Here's how the part is built. I have some questions about the finished solid (model axes, mm). A direction names the side the tool comes from. Give positions to 0.01 mm unless a question says otherwise; leave off trailing zeros. Loops run counter-clockwise (first coordinate to the right, second up) from the corner with the lowest first, then second, coordinate; pieces in that order, holes last.
Q1. Will these pins go through, and if not, where does the flat tip stop? P1, Ø4.5, axis at y = -9.5, z = 4.5, coming from the -X side; P2, Ø3, axis at y = 9, z = 2.5, coming from the +X side; P3, Ø12, axis at x = 8.5, z = 35.5, coming from the -Y side.
Q2. If we section it at C-C (x = -13.5): Please give me the cut outline in (y, z), plus the area to 3 significant figures.
Q3. We'd pull the mould along X, two halves only. Please class faces 1 (the face through (35, -17, 3)), 2 (the face through (-0.6, 5.4, 50)), 3 (the face through (-43, 0, 25)): +X half, -X half, draft (parallel to the pull), parting line (faces both ways), or undercut.
Q4. If we section it at B-B (x = -35): Please give me the cut outline in (y, z), plus the area to 3 significant figures.
Q5. If we section it at D-D (y = -7): Please give me the cut outline in (x, z), plus the area to 3 significant figures.
Q6. I need wall thicknesses on line 1 (X direction, y = -12, z = 3.95); line 2 (Y direction, x = -35, z = 3.6); line 3 (Y direction, x = 14, z = 20.5). Which ranges of each line are inside material? Lowest first, please.
Q7. If we section it at A-A (z = 14): Please give me the cut outline in (x, y), plus the area to 3 significant figures.
Q8. For faces 4 (the face through (-1, -5, 27)), 5 (the face through (-30, 10, 3)), 6 (the face through (40, 10, 3)), which set-ups out of +Z, -Z, +X, -X, +Y, -Y let a thin tool reach every point of the face, with its end or its side?
from build123d import *

# Parameters (mm, degrees)
F0_W     = 80
F0_H     = 10
F1_DEPTH = 50
F2_W     = 80
F2_H     = 10
F3_DEPTH = 5
F4_DEPTH = 6


with BuildPart() as f1:
    # F0 (on Top) → F1 (new body)
    with BuildSketch(Plane.XY):
        with BuildLine():
            ThreePointArc((43, 5), (42.12132, 7.12132), (40, 8))
            Line((40, 8), (30, 8))
            Line((30, 8), (-30, 8))
            Line((-30, 8), (-40, 8))
            ThreePointArc((-40, 8), (-42.12132, 7.12132), (-43, 5))
            Line((-43, 5), (-43, -5))
            ThreePointArc((-43, -5), (-42.12132, -7.12132), (-40, -8))
            Line((-40, -8), (-30, -8))
            Line((-30, -8), (30, -8))
            Line((30, -8), (40, -8))
            ThreePointArc((40, -8), (42.12132, -7.12132), (43, -5))
            Line((43, -5), (43, 5))
        make_face()
        Rectangle(F0_W, F0_H, mode=Mode.SUBTRACT)
    extrude(amount=F1_DEPTH)

    # F2 (on Top) → F3 (join)
    with BuildSketch(Plane.XY):
        Rectangle(F2_W, F2_H)
    extrude(amount=F3_DEPTH)

    # F0 (on Top) → F4 (join)
    with BuildSketch(Plane.XY):
        with BuildLine():
            ThreePointArc((43, 5), (42.12132, 7.12132), (40, 8))
            Line((40, 8), (30, 8))
            Line((30, 8), (-30, 8))
            Line((-30, 8), (-40, 8))
            ThreePointArc((-40, 8), (-42.12132, 7.12132), (-43, 5))
            Line((-43, 5), (-43, -5))
            ThreePointArc((-43, -5), (-42.12132, -7.12132), (-40, -8))
            Line((-40, -8), (-30, -8))
            Line((-30, -8), (30, -8))
            Line((30, -8), (40, -8))
            ThreePointArc((40, -8), (42.12132, -7.12132), (43, -5))
            Line((43, -5), (43, 5))
        make_face()
        Rectangle(F0_W, F0_H, mode=Mode.SUBTRACT)
        with BuildLine():
            Line((30, 8), (40, 8))
            Line((40, 8), (40, 12))
            Line((40, 12), (36.75, 12))
            ThreePointArc((36.75, 12), (35, 10.25), (33.25, 12))
            Line((33.25, 12), (30, 12))
            Line((30, 12), (30, 8))
        make_face()
        with BuildLine():
            Line((36.75, 12), (40, 12))
            ThreePointArc((40, 12), (35, 17), (30, 12))
            Line((30, 12), (33.25, 12))
            ThreePointArc((33.25, 12), (35, 13.75), (36.75, 12))
        make_face()
        with BuildLine():
            Line((-40, 8), (-30, 8))
            Line((-30, 8), (-30, 12))
            Line((-30, 12), (-33.25, 12))
            ThreePointArc((-33.25, 12), (-35, 10.25), (-36.75, 12))
            Line((-36.75, 12), (-40, 12))
            Line((-40, 12), (-40, 8))
        make_face()
        with BuildLine():
            Line((-33.25, 12), (-30, 12))
            ThreePointArc((-30, 12), (-35, 17), (-40, 12))
            Line((-40, 12), (-36.75, 12))
            ThreePointArc((-36.75, 12), (-35, 13.75), (-33.25, 12))
        make_face()
        with BuildLine():
            Line((40, -12), (40, -8))
            Line((40, -8), (30, -8))
            Line((30, -8), (30, -12))
            Line((30, -12), (33.25, -12))
            ThreePointArc((33.25, -12), (35, -10.25), (36.75, -12))
            Line((36.75, -12), (40, -12))
        make_face()
        with BuildLine():
            ThreePointArc((30, -12), (35, -17), (40, -12))
            Line((40, -12), (36.75, -12))
            ThreePointArc((36.75, -12), (35, -13.75), (33.25, -12))
            Line((33.25, -12), (30, -12))
        make_face()
        with BuildLine():
            Line((-30, -12), (-30, -8))
            Line((-30, -8), (-40, -8))
            Line((-40, -8), (-40, -12))
            Line((-40, -12), (-36.75, -12))
            ThreePointArc((-36.75, -12), (-35, -10.25), (-33.25, -12))
            Line((-33.25, -12), (-30, -12))
        make_face()
        with BuildLine():
            ThreePointArc((-40, -12), (-35, -17), (-30, -12))
            Line((-30, -12), (-33.25, -12))
            ThreePointArc((-33.25, -12), (-35, -13.75), (-36.75, -12))
            Line((-36.75, -12), (-40, -12))
        make_face()
    extrude(amount=F4_DEPTH)


solid = f1.part
Check sheet entries:
1. P1: stops at x = -41.98
1. P2: stops at x = 41.66
1. P3: stops at y = -8
2. outline: (-8, 0) - (8, 0) - (8, 50) - (5, 50) - (5, 5) - (-5, 5) - (-5, 50) - (-8, 50) - close
2. area: 350 mm2
3. face 1: undercut
3. face 2: draft
3. face 3: -X half
4. outline: (-17, 0) - (-13.75, 0) - (-13.75, 6) - (-17, 6) - close; (-10.25, 0) - (10.25, 0) - (10.25, 6) - (8, 6) - (8, 50) - (5, 50) - (5, 5) - (-5, 5) - (-5, 50) - (-8, 50) - (-8, 6) - (-10.25, 6) - close; (13.75, 0) - (17, 0) - (17, 6) - (13.75, 6) - close
4. area: 416 mm2
5. outline: (-42.24, 0) - (42.24, 0) - (42.24, 50) - (-42.24, 50) - close
5. area: 4,220 mm2
6. line 1: x = -40 to -36.75, -33.25 to -30, 30 to 33.25, 36.75 to 40
6. line 2: y = -17 to -13.75, -10.25 to 10.25, 13.75 to 17
6. line 3: y = -8 to -5, 5 to 8
7. outline: (-43, -5) arc R3 ccw to (-40, -8) - (40, -8) arc R3 ccw to (43, -5) - (43, 5) arc R3 ccw to (40, 8) - (-40, 8) arc R3 ccw to (-43, 5) - close; hole (-40, -5) - (40, -5) - (40, 5) - (-40, 5) - close
7. area: 568 mm2
8. face 4: +Z
8. face 5: +Z, -Z, +Y
8. face 6: +Z, -Z, +X, +Y
